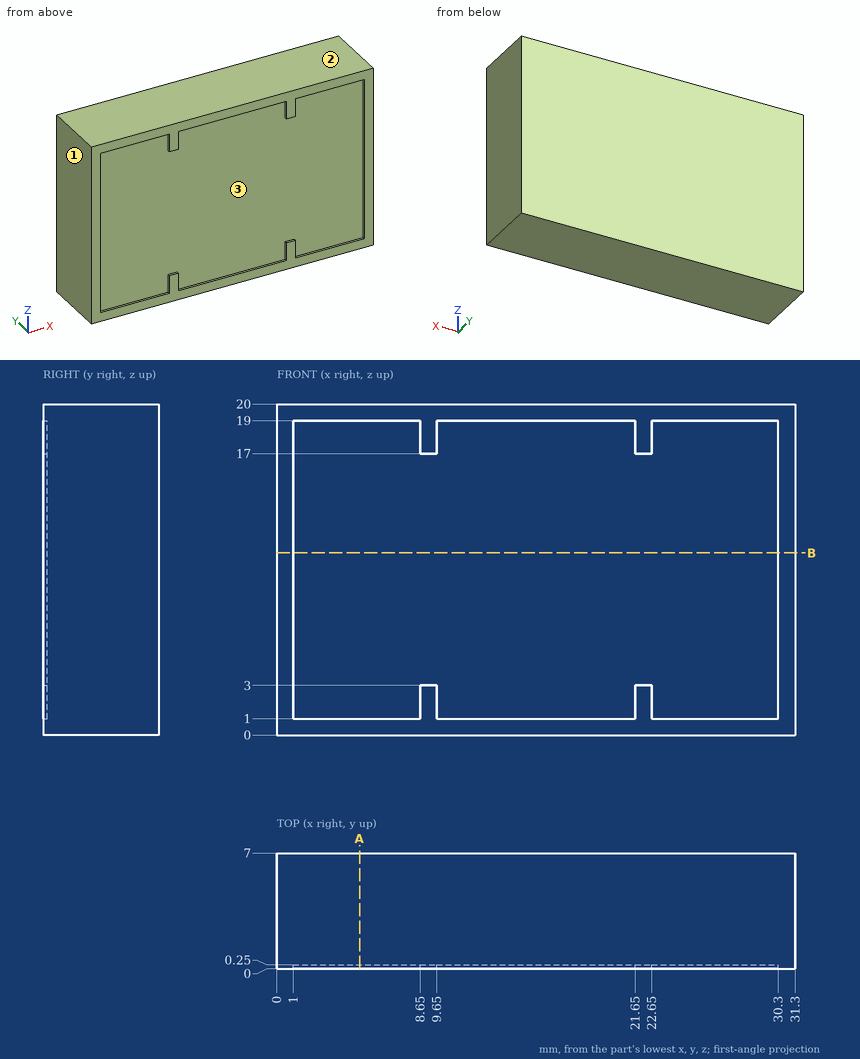
Could you check a few things on this drawing? It's one solid part, dimensions in mm from its lowest x, y, z. Coordinates: 2 decimals unless noted, no trailing zeros. Order: outer loops, then holes, each group sorted by start corner. A loop starts at its lowest first (then second) coordinate and runs counter-clockwise, first axis right, second up. Notation, with made-up numbers: (-24, -32) - (17, -32) arc R33 ccw to (17, 2) - close; hole circle Ø4 at (17, 16.5). An arc over 180 degrees is marked (long way). Answer as a JSON object with one key per item and string values. Group by question number.
Q1. Imagine slicing it at B-B (z = 11). Please give me the cut outline in (x, y), and give its area (3 significant figures).
Q2. We'd pull the mould along Z, two halves only. Please class the marked faces 1, 2 and 3: +Z half, -Z half, draft (parallel to the pull), parting line (faces both ways), or undercut.
Q3. Will this pin go through, and if not, where does the flat tip stop? P1, Ø5, axis at x = 21, z = 12, coming from the -Y side.
Q4. I need wall thicknesses on line 1 (Y direction, x = 21, z = 16.25). Which ranges of the line are inside material? Lowest first, please. Write a range as from..to.
Q5. Imagine slicing it at A-A (x = 5). Please give me the cut outline in (y, z), and give its area (4 significant figures).
Determined:
{
 "1": {"outline": "(0, 0) - (1, 0) - (1, 0.25) - (30.3, 0.25) - (30.3, 0) - (31.3, 0) - (31.3, 7) - (0, 7) - close", "area": "212 mm2"},
 "2": {"face 1": "draft", "face 2": "+Z half", "face 3": "undercut"},
 "3": {"P1": "stops at y = 0.25"},
 "4": {"line 1": "y = 0.25..7"},
 "5": {"outline": "(0, 0) - (7, 0) - (7, 20) - (0, 20) - (0, 19) - (0.25, 19) - (0.25, 1) - (0, 1) - close", "area": "135.5 mm2"}
}
